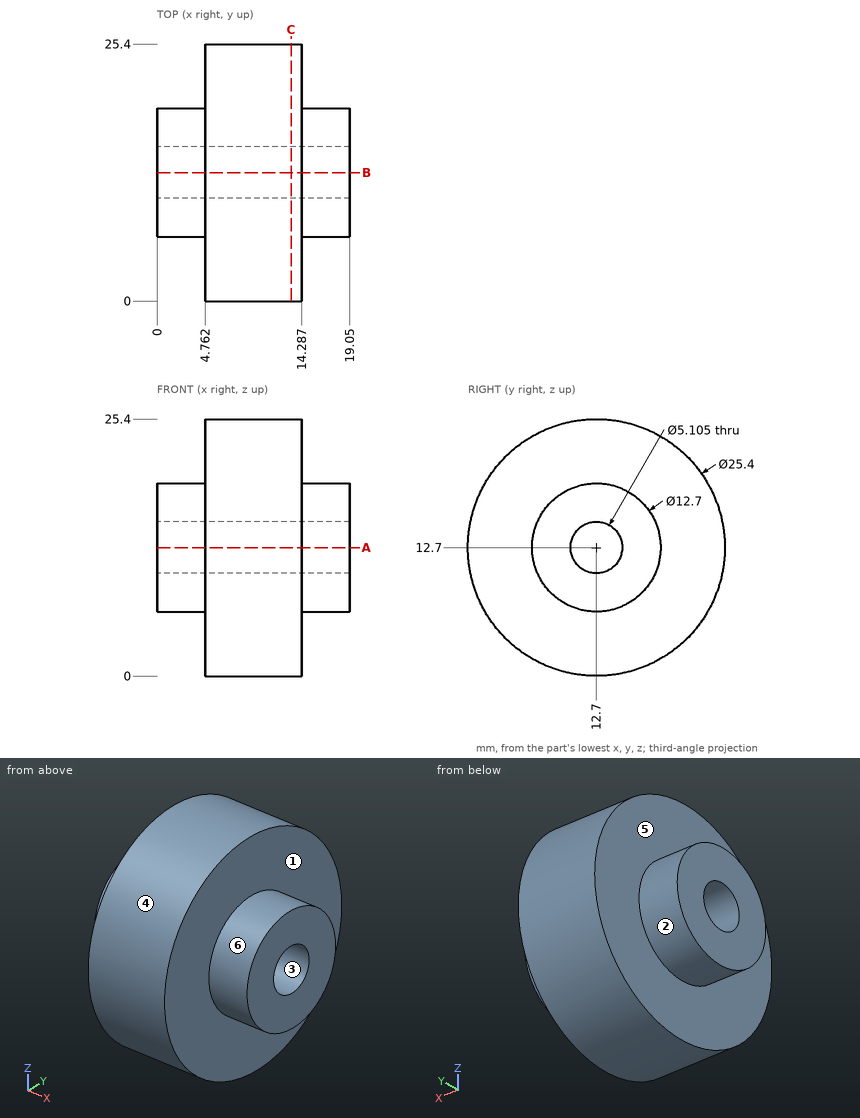
Part print with two shaded views. Sizes in mm from the minimum x, y, z corner. A direction names the side the tool comes from. Give positions to 0.01 mm unless a question says otherwise; leave off trailing zeros. Loops run counter-clockwise (first coordinate to the right, second up) from the corner with the lowest first, then second, coordinate; pieces in that order, holes last. Notation, with made-up numbers: (83, 20) -> (96, 20) arc R18 ccw to (96, 34) -> close; hole circle Ø8 at (38.5, 55.5). An arc over 180 degrees is marked (long way). One line per question, with ' | ' between items.
Q1. Cut at C-C, the plane x = 13.25. Write the cut outline in (y, z) (1 decimal), plus the area to 3 significant figures.
Filled sheet:
outline: circle Ø25.4 at (12.7, 12.7); hole circle Ø5.1 at (12.7, 12.7) | area: 486 mm²
Q2. Tool access for the marked faces 4, 5 and 6: list every direction of +Z, -Z, +X, -X, +Y, -Y with a clear straight run to the whole face (end or side of a thin tool).
Filled sheet:
face 4: +X, -X | face 5: -X | face 6: +X
Q3. Cut at A-A, the plane z = 12.7. Write the cut outline in (x, y), plus the area to 3 significant figures.
Filled sheet:
outline: (0, 6.35) -> (4.76, 6.35) -> (4.76, 0) -> (14.29, 0) -> (14.29, 6.35) -> (19.05, 6.35) -> (19.05, 10.15) -> (0, 10.15) -> close; (0, 15.25) -> (19.05, 15.25) -> (19.05, 19.05) -> (14.29, 19.05) -> (14.29, 25.4) -> (4.76, 25.4) -> (4.76, 19.05) -> (0, 19.05) -> close | area: 266 mm²
Q4. Pull direction Z, two halves, no side cores. Call the marked faces 1, 2 and 3: pulls with the +Z half, pulls with the -Z half, needs draft (parallel to the pull), parting line crosses it, or undercut.
Filled sheet:
face 1: needs draft | face 2: parting line crosses it | face 3: undercut
Q5. Drop flat-ended pins along their axis: pin 1 (8 mm diameter, centred on x = 9.5, z = 21, fed in from +Y); pin 2 (1.5 mm diameter, centred on x = 6.5, z = 19, fed in from +Y); pin 3 (1.5 mm diameter, centred on y = 6, z = 17.5, fed in from -X). Give the stop position or say it passes through.
Filled sheet:
pin 1: stops at y = 24.65 | pin 2: stops at y = 24.12 | pin 3: stops at x = 4.76
Q6. Drill centre lines: line 1 along Y through (x, z) = (14.75, 12.7); line 2 along Z through (x, y) = (6.25, 12.75). Where is each one in solid material? Low to high. Write a range as [from, to].
Filled sheet:
line 1: y = [6.35, 10.15], [15.25, 19.05] | line 2: z = [0, 10.15], [15.25, 25.4]
